Model file for the job. Use its own axes, mm. A direction names the side the tool comes from. Coordinates: 2 decimals unless noted, no trailing zeros. Order: outer loops, then holes, each group sorted by start corner. A loop starts at its lowest first (then second) coordinate and runs counter-clockwise, first axis right, second up.
from build123d import *

# Parameters (mm, degrees)
SKETCH1_W                   = 50
SKETCH1_H                   = 110
BOSS_EXTRUDE1_DEPTH         = 10
FILLET1_R                   = 10
SKETCH3_W                   = 50
SKETCH3_H                   = 50
BOSS_EXTRUDE2_DEPTH         = 60
SKETCH4_R                   = 14
BOSS_EXTRUDE3_DEPTH         = 12
SKETCH5_R                   = 12
BOSS_EXTRUDE4_DEPTH         = 20
HOLE1_D                     = 10
HOLE1_CBORE_D               = 20
HOLE1_CBORE_DEPTH           = 2
HOLE2_D                     = 14
HOLE2_CBORE_D               = 33
HOLE2_CBORE_DEPTH           = 44
M33X2_0_TAPPED_HOLE1_REACH  = 124.07
M33X2_0_TAPPED_HOLE1_BORE_R = 15.5
HOLE4_D                     = 18
HOLE4_CBORE_D               = 30
HOLE4_CBORE_DEPTH           = 22
CHAMFER3_SIZE               = 2


with BuildPart() as part:
    # Sketch1 → Boss-Extrude1 (new body)
    with BuildSketch(Plane(origin=(0, 0, 0), x_dir=(0, 1, 0), z_dir=(0, 0, 1))):
        Rectangle(SKETCH1_W, SKETCH1_H)
    extrude(amount=BOSS_EXTRUDE1_DEPTH)

    # Fillet1
    fillet1_edges = [part.edges().sort_by_distance(p)[0] for p in [
        (55, 25, 5),
        (55, -25, 5),
        (-55, -25, 5),
        (-55, 25, 5),
    ]]
    fillet(fillet1_edges, radius=FILLET1_R)

    # Sketch3 → Boss-Extrude2 (add)
    with BuildSketch(Plane(origin=(0, 0, 0), x_dir=(0, 1, 0), z_dir=(0, 0, 1))):
        Rectangle(SKETCH3_W, SKETCH3_H)
    extrude(amount=BOSS_EXTRUDE2_DEPTH)

    # Sketch4 → Boss-Extrude3 (add)
    with BuildSketch(Plane(origin=(0, 0, 0), x_dir=(1, 0, 0), z_dir=(0, 0, -1))):
        with Locations(Location((0, 0, 0), (0, 0, 180))):
            Circle(SKETCH4_R)
    extrude(amount=BOSS_EXTRUDE3_DEPTH)

    # Sketch5 → Boss-Extrude4 (add)
    with BuildSketch(Plane(origin=(0, 0, 0), x_dir=(1, 0, 0), z_dir=(0, 0, -1))):
        with Locations(Location((0, 0, 0), (0, 0, 180))):
            Circle(SKETCH5_R)
    extrude(amount=BOSS_EXTRUDE4_DEPTH)

    # Sketch7 → Revolve1 (revolve)
    with BuildSketch(Plane(origin=(0, 0, 30), x_dir=(0, 1, 0), z_dir=(0, 0, 1)), mode=Mode.PRIVATE) as revolve1_sk:
        Polygon((25, 17.5), (43, 17.5), (43, 13.5), (54, 13.5), (54, 11.5), (57, 11.5), (57, 13.5), (74, 13.5), (74, 0), (25, 0), align=None)
    revolve(revolve1_sk.sketch.rotate(Axis((0, 0, 30), (0, 1, 0)), 270), axis=Axis((0, 0, 30), (0, 1, 0)))

    # Hole1 (through all)
    with Locations(Plane.XY.offset(10)):
        with Locations((-45, -15), (-45, 15)):
            hole1 = CounterBoreHole(HOLE1_D / 2, HOLE1_CBORE_D / 2, HOLE1_CBORE_DEPTH)

    # Mirror1: Hole1 across plane
    add(hole1.mirror(Plane(origin=(0, 0, 0), x_dir=(0, 0, 1), z_dir=(1, 0, 0))), mode=Mode.SUBTRACT)

    # Sketch12 → Revolve2 (revolve)
    with BuildSketch(Plane(origin=(0, 0, 30), x_dir=(0, 1, 0), z_dir=(0, 0, 1))):
        with BuildLine():
            Line((-25, 35), (-10, 35))
            ThreePointArc((-10, 35), (-2.928932188, 32.071067812), (0, 25))
            Line((0, 25), (-25, 25))
            Line((-25, 25), (-25, 35))
        make_face()
    revolve2 = revolve(axis=Axis((-25, 0, 30), (0, -1, 0)))

    # Mirror2: Revolve2 across plane
    add(revolve2.mirror(Plane(origin=(0, 0, 0), x_dir=(0, 0, 1), z_dir=(1, 0, 0))))

    # Hole2 (through all)
    with Locations(Plane.XZ.offset(25)):
        with Locations((0, 30)):
            CounterBoreHole(HOLE2_D / 2, HOLE2_CBORE_D / 2, HOLE2_CBORE_DEPTH)

    # Sketch16 → M10 Tapped Hole1 (revolve, cut)
    with BuildSketch(Plane(origin=(-25, -25, 30), x_dir=(0, 0, -1), z_dir=(1, 0, 0))):
        Polygon((0, 0), (0, 17.553657631), (4.25, 15), (4.25, 0), align=None)
    m10_tapped_hole1 = revolve(axis=Axis((-25, -31.35, 30), (0, 1, 0)), mode=Mode.SUBTRACT)

    # Mirror4: M10 Tapped Hole1 across plane
    add(m10_tapped_hole1.mirror(Plane(origin=(0, 0, 0), x_dir=(0, 0, 1), z_dir=(1, 0, 0))), mode=Mode.SUBTRACT)

    # M33x2.0 Tapped Hole1 bore → M33x2.0 Tapped Hole1 (cut, up to next)
    with BuildSketch(Plane.XY.offset(60), mode=Mode.PRIVATE) as m33x2_0_tapped_hole1_sk1:
        Circle(M33X2_0_TAPPED_HOLE1_BORE_R)
    m33x2_0_tapped_hole1_tool1 = extrude(m33x2_0_tapped_hole1_sk1.sketch, amount=-M33X2_0_TAPPED_HOLE1_REACH, mode=Mode.PRIVATE) & part.part
    add(m33x2_0_tapped_hole1_tool1.solids().sort_by_distance((0, 0, 60))[0], mode=Mode.SUBTRACT)

    # Hole4 (through all)
    with Locations(Plane(origin=(0, 0, 30), x_dir=(0, 1, 0), z_dir=(0, 0, 1))):
        with Locations((0, 0)):
            CounterBoreHole(HOLE4_D / 2, HOLE4_CBORE_D / 2, HOLE4_CBORE_DEPTH)

    # Chamfer3
    chamfer3_edges = [part.edges().sort_by_distance(p)[0] for p in [
        (-16.5, -25, 30),
        (-15.5, 0, 60),
        (14, 0, -12),
        (12, 0, -20),
        (0, 43, 47.5),
        (0, 74, 43.5),
    ]]
    chamfer(chamfer3_edges, length=CHAMFER3_SIZE - 0.0001)  # a hair under: the kernel refuses the full size


solid = part.part
Q1. Drop flat-ended pins along their axis: P1, Ø21.5, axis at x = -5.5, z = 30, coming from the -Y side; P2, Ø8, axis at x = 45, y = -15, coming from the -Z side; P3, Ø1.5, axis at x = -2.5, y = 16.5, coming from the +Z side; P4, Ø16, axis at x = 45, y = 15, coming from the +Z side. Give the stop position or say it passes through.
Established:
P1: stops at y = 19
P2: passes through
P3: stops at z = 59.94
P4: stops at z = 8
Q2. Cut at A-A, the plane y = 27.5. List the corners of the cut face in (x, z), plus the area to 3 significant figures.
Established:
outline: circle Ø35 at (0, 30); hole circle Ø14 at (0, 30)
area: 808 mm2
Q3. Which spindle directions (+Z, -Z, +X, -X, +Y, -Y) get a long thin tool onto all of the face, cutting with end or side? Do faces 4 (the face through (25.187, -17.605, 34.246)), 5 (the face through (50, 13, 8)), 6 (the face through (-13, 43, 35)). Say none if no direction does.
Established:
face 4: -Y
face 5: +Z
face 6: +Y
Q4. Probe line 1 (Y direction, x = 45, z = 5.5); line 2 (X direction, y = 0, z = 45); line 3 (Y direction, x = -17.5, z = 14). List the from-to ranges inside material, lowest first.
Established:
line 1: y = -25 to -20, -10 to 10, 20 to 25
line 2: x = -25 to -15.5, 15.5 to 25
line 3: y = -25 to 25
Q5. Cut at B-B, the plane y = 68. List the corners of the cut face in (x, z).
Established:
outline: circle Ø27 at (0, 30); hole circle Ø14 at (0, 30)
Q6. Mould opens along Z. For faces 1 (the face through (-35, -17, 30)), 2 (the face through (-6, 54, 20)), 3 (the face through (-0.51, 55.52, 41.49)) say: pulls with the +Z half, pulls with the -Z half, needs draft (parallel to the pull), parting line crosses it, or undercut.
Established:
face 1: undercut
face 2: needs draft
face 3: parting line crosses it
